Geometry check sheet. Reference: the model listing, model coordinates, mm. A direction names the side the tool comes from. Coordinates: 2 decimals unless noted, no trailing zeros. Write each loop counter-clockwise with the first axis right and the second up, starting at its lowest first coordinate (ties: lowest second). Pieces come first, ordered by that corner, then holes. Notation, with made-up numbers: M 25,78 L 69,78 A16 ccw 69,84 Z; hole C 33.25,-24 d10. An arc over 180 degrees is marked long. Answer as a JSON object with one key per item and string values. Group by question number.
```python
from build123d import *

# Parameters (mm, degrees)
SKETCH1_R           = 8.89
SKETCH1_R_2         = 1.016
BOSS_EXTRUDE1_DEPTH = 0.5
CUT_EXTRUDE1_DEPTH  = 0.5
BOSS_EXTRUDE2_START = 1
SKETCH3_R           = 1.216
SKETCH3_R_2         = 1.016
BOSS_EXTRUDE2_DEPTH = 1
FILLET1_R           = 1


with BuildPart() as part:
    # Sketch1 → Boss-Extrude1 (new body)
    with BuildSketch(Plane.XY):
        Circle(SKETCH1_R)
        Circle(SKETCH1_R_2, mode=Mode.SUBTRACT)
    extrude(amount=-BOSS_EXTRUDE1_DEPTH)

    # Sketch2 → Cut-Extrude1 (cut)
    with BuildSketch(Plane.XY):
        with BuildLine():
            ThreePointArc((-2.388296759, 3.748874977), (-1.61103708, 4.142774979), (-0.77186615, 4.377470462))
            Line((-0.77186615, 4.377470462), (-1.543732299, 8.754940924))
            ThreePointArc((-1.543732299, 8.754940924), (-3.22207416, 8.285549958), (-4.776593518, 7.497749953))
            Line((-4.776593518, 7.497749953), (-2.388296759, 3.748874977))
        make_face()
        with BuildLine():
            ThreePointArc((5.099094519, 7.282261674), (3.580418073, 8.137119049), (1.924148168, 8.679271503))
            Line((1.924148168, 8.679271503), (0.962074084, 4.339635752))
            ThreePointArc((0.962074084, 4.339635752), (1.790209036, 4.068559525), (2.54954726, 3.641130837))
            Line((2.54954726, 3.641130837), (5.099094519, 7.282261674))
        make_face()
        with BuildLine():
            ThreePointArc((8.754940924, 1.543732299), (8.285549958, 3.22207416), (7.497749953, 4.776593518))
            Line((7.497749953, 4.776593518), (3.748874977, 2.388296759))
            ThreePointArc((3.748874977, 2.388296759), (4.142774979, 1.61103708), (4.377470462, 0.77186615))
            Line((4.377470462, 0.77186615), (8.754940924, 1.543732299))
        make_face()
        with BuildLine():
            ThreePointArc((7.282261674, -5.099094519), (8.137119049, -3.580418073), (8.679271503, -1.924148168))
            Line((8.679271503, -1.924148168), (4.339635752, -0.962074084))
            ThreePointArc((4.339635752, -0.962074084), (4.068559525, -1.790209036), (3.641130837, -2.54954726))
            Line((3.641130837, -2.54954726), (7.282261674, -5.099094519))
        make_face()
        with BuildLine():
            ThreePointArc((1.543732299, -8.754940924), (3.22207416, -8.285549958), (4.776593518, -7.497749953))
            Line((4.776593518, -7.497749953), (2.388296759, -3.748874977))
            ThreePointArc((2.388296759, -3.748874977), (1.61103708, -4.142774979), (0.77186615, -4.377470462))
            Line((0.77186615, -4.377470462), (1.543732299, -8.754940924))
        make_face()
        with BuildLine():
            Line((-2.54954726, -3.641130837), (-5.099094519, -7.282261674))
            ThreePointArc((-5.099094519, -7.282261674), (-3.580418073, -8.137119049), (-1.924148168, -8.679271503))
            Line((-1.924148168, -8.679271503), (-0.962074084, -4.339635752))
            ThreePointArc((-0.962074084, -4.339635752), (-1.790209036, -4.068559525), (-2.54954726, -3.641130837))
        make_face()
        with BuildLine():
            Line((-4.377470462, -0.77186615), (-8.754940924, -1.543732299))
            ThreePointArc((-8.754940924, -1.543732299), (-8.285549958, -3.22207416), (-7.497749953, -4.776593518))
            Line((-7.497749953, -4.776593518), (-3.748874977, -2.388296759))
            ThreePointArc((-3.748874977, -2.388296759), (-4.142774979, -1.61103708), (-4.377470462, -0.77186615))
        make_face()
        with BuildLine():
            Line((-3.641130837, 2.54954726), (-7.282261674, 5.099094519))
            ThreePointArc((-7.282261674, 5.099094519), (-8.137119049, 3.580418073), (-8.679271503, 1.924148168))
            Line((-8.679271503, 1.924148168), (-4.339635752, 0.962074084))
            ThreePointArc((-4.339635752, 0.962074084), (-4.068559525, 1.790209036), (-3.641130837, 2.54954726))
        make_face()
    extrude(amount=-CUT_EXTRUDE1_DEPTH, mode=Mode.SUBTRACT)

    # Sketch3 → Boss-Extrude2 (add)
    with BuildSketch(Plane.XY.offset(BOSS_EXTRUDE2_START)):
        Circle(SKETCH3_R)
        Circle(SKETCH3_R_2, mode=Mode.SUBTRACT)
    extrude(amount=-BOSS_EXTRUDE2_DEPTH)

    # Fillet1
    fillet1_edges = [part.edges().sort_by_distance(p)[0] for p in [
        (-1.216, 0, 0),
    ]]
    fillet(fillet1_edges, radius=FILLET1_R - 0.0001)  # a hair under: the kernel refuses the full size


solid = part.part
```
1) Section check D-D (z = 0.6). Record the cut outline in (x, y), then the cut area to 3 significant figures.
2) Material ranges on probe 1 along Y at (x, z) = (5, -0.3); probe 2 along Y at (x, z) = (0, -0.2); probe 3 along Z at (x, y) = (1.25, -2), recorded low to high. Write a range as [from, to].
3) Section check C-C (y = 3). Record the cut outline in (x, z).
4) Set-up check for faces 5 (the flat face through (5.44, -3.81, -0.25)), 6 (the flat face through (-3.6, 5.65, -0.25)), 7 (the flat face through (-5.65, -3.6, -0.25)), 8 (the flat face through (-1.45, -6.54, -0.25)), 9 (the flat face through (-3.81, -5.44, -0.25)): record each of +Z, -Z, +X, -X, +Y, -Y from which the full face is reachable in a straight line by a thin tool's end or side.
5) Draft check along Y on faces 1 (the cylindrical face through (-6.13, 6.44, -0.25)), 2 (the flat face through (2, -2, 0)), 3 (the flat face through (1.45, 6.54, -0.25)), 4 (the flat face through (5.65, 3.6, -0.25)). Enter one of: +Y half, -Y half, draft (parallel to the pull), parting line (faces both ways), or undercut.
Entries:
{
 "1": {"outline": "C 0,0 d2.6; hole C 0,0 d2.03", "area": "2.06 mm^2"},
 "2": {"probe 1": "[-7.35, -3.5], [-1.11, 0.88], [3.19, 7.14]", "probe 2": "[-8.89, -1.02], [1.02, 8.89]", "probe 3": "[-0.5, 0]"},
 "3": {"outline": "M -4.28,-0.5 L 4.71,-0.5 L 4.71,0 L -4.28,0 Z"},
 "4": {"face 5": "+Z, -Z, +X", "face 6": "+Z, -Z, +Y", "face 7": "+Z, -Z, -X", "face 8": "+Z, -Z", "face 9": "+Z, -Z, -Y"},
 "5": {"face 1": "+Y half", "face 2": "draft", "face 3": "undercut", "face 4": "undercut"}
}
